CAD build for the part. Positions are in the model's coordinates, mm. Face numbers are marked on the shaded views. A direction names the side the tool comes from. Round coordinates to 2 decimals unless told otherwise and drop trailing zeros. Loops run counter-clockwise (first coordinate to the right, second up) from the corner with the lowest first, then second, coordinate; pieces in that order, holes last. Notation, with made-up numbers: (-22.5, 7) - (0.5, 7) arc R21 cw to (0.5, 35) - close; hole circle Ø11 at (-7.5, 50). An arc over 180 degrees is marked (long way). One line per question, with ' | ' between items.
```python
from build123d import *

# Parameters (mm, degrees)
AUFSATZ_LINEAR_AUSTRAGEN1_DEPTH       = 90
AUFSATZ_LINEAR_AUSTRAGEN1_DEPTH_BACK  = 0.0001
SCHNITT_LINEAR_AUSTRAGEN1_DEPTH       = 80
AUFSATZ_LINEAR_START                  = -10.0001
AUFSATZ_LINEAR_AUSTRAGEN2_DEPTH       = 10.0001
SKIZZE45_R                            = 2.25
SCHNITT_LINEAR_AUSTRAGEN9_DEPTH       = 5
SCHNITT_LINEAR_AUSTRAGEN16_DEPTH      = 101.498845765
SCHNITT_LINEAR_AUSTRAGEN16_DEPTH_BACK = 101.498845765
F_2_5_2_5_DURCHMESSER_BOHRUNG1_D      = 2.5


# Read off the part's stored shape, not the designer's step: Aufsatz-Linear austragen2
with BuildPart() as part:
    # Skizze1 → Aufsatz-Linear austragen1 (new, two sides: drawn at the far end of the back side and taken through both)
    with BuildSketch(Plane(origin=(0, 0, 0), x_dir=(1, 0, 0), z_dir=(0, 1, 0)).offset(-AUFSATZ_LINEAR_AUSTRAGEN1_DEPTH_BACK)):
        with BuildLine():
            Line((0, 0), (40, 0))
            ThreePointArc((40, 0), (20, 20), (0, 0))
        make_face()
    extrude(amount=AUFSATZ_LINEAR_AUSTRAGEN1_DEPTH + AUFSATZ_LINEAR_AUSTRAGEN1_DEPTH_BACK)

    # Skizze15 → Schnitt-Linear austragen1 (cut)
    with BuildSketch(Plane(origin=(0, 90, 0), x_dir=(1, 0, 0), z_dir=(0, 1, 0))):
        with BuildLine():
            Line((25, 0), (15, 0))
            ThreePointArc((15, 0), (20, 5), (25, 0))
        make_face()
    extrude(amount=-SCHNITT_LINEAR_AUSTRAGEN1_DEPTH, mode=Mode.SUBTRACT)

    # Aufsatz-Linear austragen2 outline → Aufsatz-Linear austragen2 (cut)
    with BuildSketch(Plane(origin=(0, 10, 0), x_dir=(1, 0, 0), z_dir=(0, 1, 0)).offset(AUFSATZ_LINEAR_START)):
        with BuildLine():
            Line((19, 0), (21, 0))
            ThreePointArc((21, 0), (20, 1), (19, 0))
        make_face()
    extrude(amount=AUFSATZ_LINEAR_AUSTRAGEN2_DEPTH, mode=Mode.SUBTRACT)

    # Skizze45 → Schnitt-Linear austragen9 (cut)
    with BuildSketch(Plane.XZ.offset(0.0001)):
        with Locations((20, 0)):
            Circle(SKIZZE45_R)
    extrude(amount=-SCHNITT_LINEAR_AUSTRAGEN9_DEPTH, mode=Mode.SUBTRACT)

    # Skizze47 → Schnitt-Linear austragen16 (cut, two sides: drawn at the far end of the back side and taken through both)
    with BuildSketch(Plane.XZ.offset(0.0001).offset(-SCHNITT_LINEAR_AUSTRAGEN16_DEPTH_BACK)):
        Polygon((-96.877045312, -2.5), (0.156865167, -2.5), (12.5, -2.5), (12.5, -8.61), (27.5, -8.61), (27.5, -2.5), (39.843134833, -2.5), (136.877045312, -2.5), (136.877045312, -196.567820958), (-96.877045312, -196.567820958), align=None)
    extrude(amount=SCHNITT_LINEAR_AUSTRAGEN16_DEPTH + SCHNITT_LINEAR_AUSTRAGEN16_DEPTH_BACK, mode=Mode.SUBTRACT)

    # Ø2.5 (2.5) Durchmesser Bohrung1 (through all)
    with Locations(Plane.XY):
        with Locations((6, 75), (6, 15), (34, 75), (34, 15)):
            Hole(F_2_5_2_5_DURCHMESSER_BOHRUNG1_D / 2)


solid = part.part
```
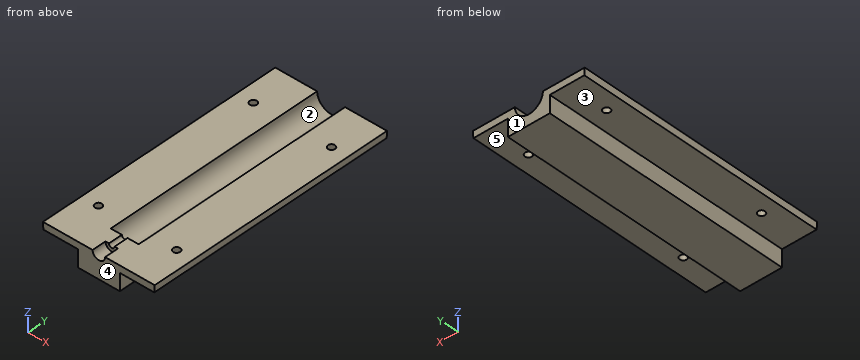
(1) Two-plate mould, pull along X, no slides. Class the marked faces 1 and 2: released by +X, released by -X, zero draft, split by the parting line, or undercut.
Results found:
face 1: zero draft | face 2: undercut
(2) Cut at C-C, the plane y = 42. Write the cut outline in (x, z).
Results found:
outline: (0, 0) arc R20 ccw to (0.16, -2.5) - (12.5, -2.5) - (12.5, -8.61) - (27.5, -8.61) - (27.5, -2.5) - (39.84, -2.5) arc R20 ccw to (40, 0) - (25, 0) arc R5 cw to (15, 0) - close
(3) Cut at A-A, the plane x = 6. Write the cut outline in (y, z), then the cut area to 4 significant figures.
Results found:
outline: (0, -2.5) - (13.75, -2.5) - (13.75, 0) - (0, 0) - close; (16.25, -2.5) - (73.75, -2.5) - (73.75, 0) - (16.25, 0) - close; (76.25, -2.5) - (90, -2.5) - (90, 0) - (76.25, 0) - close | area: 212.5 mm²
(4) Cut at D-D, the plane x = 20. Write the cut outline in (y, z), then the cut area to 3 significant figures.
Results found:
outline: (0, -8.61) - (90, -8.61) - (90, -5) - (10, -5) - (10, -1) - (5, -1) - (5, -2.25) - (0, -2.25) - close | area: 359 mm²
(5) Tool access for the marked faces 3, 4 and 5: list every direction of +Z, -Z, +X, -X, +Y, -Y with a clear straight run to the whole face (end or side of a thin tool).
Results found:
face 3: -Z, -X, +Y, -Y | face 4: +Z, -Z, +X, -X, -Y | face 5: -Z, +X, +Y, -Y
(6) Cut at B-B, the plane y = 75. Write the cut outline in (x, z), then the cut area to 3 significant figures.
Results found:
outline: (0, 0) arc R20 ccw to (0.16, -2.5) - (4.75, -2.5) - (4.75, 0) - close; (7.25, -2.5) - (12.5, -2.5) - (12.5, -8.61) - (27.5, -8.61) - (27.5, -2.5) - (32.75, -2.5) - (32.75, 0) - (25, 0) arc R5 cw to (15, 0) - (7.25, 0) - close; (35.25, -2.5) - (39.84, -2.5) arc R20 ccw to (40, 0) - (35.25, 0) - close | area: 140 mm²
(7) Probe L1, parallel to Y at x = 34, z = -1.05; L2, parallel to Y at x = 5, z = -1; L3, parallel to X at y = 75, z = -1.8. List the from-to ranges inside material, lowest first.
Results found:
L1: y = 0 to 13.75, 16.25 to 73.75, 76.25 to 90 | L2: y = 0 to 14.25, 15.75 to 74.25, 75.75 to 90 | L3: x = 0.08 to 4.75, 7.25 to 15.34, 24.66 to 32.75, 35.25 to 39.92
(8) Drop flat-ended pins along their axis: P1, Ø1.5, axis at x = 6, y = 15, coming from the -Z side; P2, Ø2, axis at x = 23.5, y = 28, coming from the +Z side; P3, Ø13.5, axis at x = 35.5, y = 31, coming from the -Z side; P4, Ø5, axis at y = 52, z = -6, coming from the +X side. Give the stop position or say it passes through.
Results found:
P1: passes through | P2: stops at z = -2.18 | P3: stops at z = -2.5 | P4: stops at x = 27.5
